Here's how the part is built. I have some questions about the finished solid (model axes, mm). A direction names the side the tool comes from. Give positions to 0.01 mm unless a question says otherwise; leave off trailing zeros. Loops run counter-clockwise (first coordinate to the right, second up) from the corner with the lowest first, then second, coordinate; pieces in that order, holes last. Notation, with made-up numbers: (-16.75, 8.5) - (6.25, 8.5) arc R24 cw to (6.25, 18.5) - close; hole circle Ø9 at (67.25, 31.25). An arc over 180 degrees is marked (long way). Use a Markdown table: item, result.
from build123d import *
from build123d.topology import SkipClean

# Parameters (mm, degrees)
SKETCH1_R           = 4.05
BOSS_EXTRUDE1_DEPTH = 5
SCALE1_SCALE        = 0.471698113
SKETCH2_R           = 1.910377358
BOSS_EXTRUDE3_DEPTH = 4.716981
SKETCH3_R           = 9.5
CUT_EXTRUDE1_DEPTH  = 35.525365892
SKETCH4_R           = 13.5
CUT_EXTRUDE2_DEPTH  = 35.525365892
SKETCH5_R           = 1.5
CUT_EXTRUDE3_DEPTH  = 35.525365892
FILLET1_R           = 5
BOSS_EXTRUDE4_START = 5
SKETCH6_R           = 9.5
SKETCH6_R_2         = 1.5
BOSS_EXTRUDE4_DEPTH = 5


with BuildPart() as part:
    # Sketch1 → Boss-Extrude1 (new, symmetric)
    with BuildSketch(Plane(origin=(0, 0, 0), x_dir=(1, 0, 0), z_dir=(0, 1, 0))):
        with BuildLine():
            Line((-38, 7.05), (38, 7.05))
            ThreePointArc((38, 7.05), (45.05, 0), (38, -7.05))
            Line((38, -7.05), (-38, -7.05))
            ThreePointArc((-38, -7.05), (-45.05, 0), (-38, 7.05))
        make_face()
        with Locations(Location((-38, 0, 0), (0, 0, 270))):
            Circle(SKETCH1_R, mode=Mode.SUBTRACT)
        with Locations(Location((38, 0, 0), (0, 0, 270))):
            Circle(SKETCH1_R, mode=Mode.SUBTRACT)
    extrude(amount=BOSS_EXTRUDE1_DEPTH, both=True)


with BuildPart() as part_1:
    # Scale1: scaled about (0, 0, 0)
    add(part.part.scale(SCALE1_SCALE))

    # Sketch2 → Boss-Extrude3 (add, through all)
    with BuildSketch(Plane(origin=(0, 2.358490566, 0), x_dir=(1, 0, 0), z_dir=(0, 1, 0))):
        with BuildLine():
            Line((8.163095128, 9.325471698), (-8.163095128, 9.325471698))
            ThreePointArc((-8.163095128, 9.325471698), (-31.424528302, 0), (-8.163095128, -9.325471698))
            Line((-8.163095128, -9.325471698), (8.163095128, -9.325471698))
            ThreePointArc((8.163095128, -9.325471698), (31.424528302, 0), (8.163095128, 9.325471698))
        make_face()
        with Locations(Location((-17.924528302, 0, 0), (0, 0, 270))):
            Circle(SKETCH2_R, mode=Mode.SUBTRACT)
        with Locations(Location((17.924528302, 0, 0), (0, 0, 270))):
            Circle(SKETCH2_R, mode=Mode.SUBTRACT)
    extrude(amount=-BOSS_EXTRUDE3_DEPTH)

    # Sketch3 → Cut-Extrude1 (cut, through all)
    with BuildSketch(Plane(origin=(0, 2.358490566, 0), x_dir=(1, 0, 0), z_dir=(0, 1, 0))):
        with Locations(Location((-17.924528302, 0, 0), (0, 0, 270))):
            Circle(SKETCH3_R)
        with Locations(Location((17.924528302, 0, 0), (0, 0, 270))):
            Circle(SKETCH3_R)
    extrude(amount=-CUT_EXTRUDE1_DEPTH, mode=Mode.SUBTRACT)

    # Sketch4 → Cut-Extrude2 (cut, through all)
    with BuildSketch(Plane(origin=(0, 2.358490566, 0), x_dir=(1, 0, 0), z_dir=(0, 1, 0))):
        with Locations((17.924528302, 0)):
            Circle(SKETCH4_R)
    extrude(amount=-CUT_EXTRUDE2_DEPTH, mode=Mode.SUBTRACT)

    # Sketch5 → Cut-Extrude3 (cut, through all)
    with BuildSketch(Plane(origin=(0, 2.358490566, 0), x_dir=(1, 0, 0), z_dir=(0, 1, 0))):
        with Locations(Location((0, 6.325471698, 0), (0, 0, 270))):
            Circle(SKETCH5_R)
        with Locations(Location((0, -6.325471698, 0), (0, 0, 270))):
            Circle(SKETCH5_R)
    extrude(amount=-CUT_EXTRUDE3_DEPTH, mode=Mode.SUBTRACT)

    # Fillet1
    # the kernel refuses this fillet: 5 mm, written as the material it takes off along each edge
    with BuildSketch(Plane(origin=(8.163095128, 22.922972313, -9.325471698), x_dir=(-0.47879135569736214, 0, 0.8779287201757795), z_dir=(0, -1, 0))) as fillet1_piece_1:
        with BuildLine():
            CenterArc((8.328082039, 4.827702878), FILLET1_R, 151.393506733, 103.521444362)
            Line((3.938438438, 7.221659656), (0, 0))
            ThreePointArc((0, 0), (3.51340961, 0.46520223), (7.02681922, 0))
        make_face()
    extrude(amount=45.845944493, mode=Mode.SUBTRACT)
    with BuildSketch(Plane(origin=(8.163095128, 22.922972313, 9.325471698), x_dir=(-1, 0, 0), z_dir=(0, -1, 0))) as fillet1_piece_2:
        with BuildLine():
            CenterArc((8.225792699, 5), FILLET1_R, 166.478555638, 103.521444362)
            ThreePointArc((3.364380301, 6.169046405), (2.090604549, 2.861788396), (0, 0))
            Line((0, 0), (8.225792699, 0))
        make_face()
    extrude(amount=45.845944493, mode=Mode.SUBTRACT)

    # Sketch6 → Boss-Extrude4 (add)
    with SkipClean():  # the faces are left unmerged after this step: merging them gives an invalid solid
        with BuildSketch(Plane(origin=(0, -2.358490566, 0), x_dir=(1, 0, 0), z_dir=(0, 1, 0)).offset(BOSS_EXTRUDE4_START)):
            with BuildLine():
                Line((-8.163095128, -9.325471698), (-0.062697571, -9.325471698))
                ThreePointArc((-0.062697571, -9.325471698), (3.864466293, -7.42020658), (4.798714827, -3.156425293))
                ThreePointArc((4.798714827, -3.156425293), (4.424528302, 0), (4.798714827, 3.156425293))
                ThreePointArc((4.798714827, 3.156425293), (3.864466293, 7.42020658), (-0.062697571, 9.325471698))
                Line((-0.062697571, 9.325471698), (-8.163095128, 9.325471698))
                ThreePointArc((-8.163095128, 9.325471698), (-31.424528302, 0), (-8.163095128, -9.325471698))
            make_face()
            with Locations(Location((-17.924528302, 0, 0), (0, 0, 270))):
                Circle(SKETCH6_R, mode=Mode.SUBTRACT)
            with Locations(Location((0, -6.325471698, 0), (0, 0, 270))):
                Circle(SKETCH6_R_2, mode=Mode.SUBTRACT)
            with Locations(Location((0, 6.325471698, 0), (0, 0, 270))):
                Circle(SKETCH6_R_2, mode=Mode.SUBTRACT)
        extrude(amount=-BOSS_EXTRUDE4_DEPTH)
    add(part_1.part.scale(1), mode=Mode.REPLACE)  # the faces are merged on a copy


solid = part_1.part
(1) On a 3-axis mill with a long thin cutter (end or side, diameter ignored), from which of +Z, -Z, +X, -X, +Y, -Y can I reach the whole of each face in a straight line? I mean faces 1 (the face through (-4, 0, 9.325)), 2 (the face through (-9, 2.642, 6)). Say none if no direction works.
A:
| item | result |
|---|---|
| face 1 | +Z, +X, +Y, -Y |
| face 2 | +Z, -Z, +X, -X, +Y |
(2) If I drill on line 1 (X direction, y = -0.3, z = 0); line 2 (Z direction, x = 1, y = -0.6); line 3 (X direction, y = 1.2, z = 8.25), over which ranges is the centre line in solid material (lowest first)?
A:
| item | result |
|---|---|
| line 1 | -31.42 to -27.42, -8.42 to 4.42 |
| line 2 | -9.21 to -7.44, -5.21 to 5.21, 7.44 to 9.21 |
| line 3 | -28.61 to -22.63, -13.21 to 3.04 |
(3) Will these pins go through, and if not, where does the flat tip stop? pin 1 (1 mm diameter, centred on x = -22, y = -1.5, fed in from +Z); pin 2 (2 mm diameter, centred on y = 0.5, z = -0.5, fed in from +X); pin 3 (1.5 mm diameter, centred on y = 0, z = 1.5, fed in from -X).
A:
| item | result |
|---|---|
| pin 1 | z = 13.02 |
| pin 2 | x = 4.51 |
| pin 3 | x = -31.4 |
(4) Suppose I cut it at D-D on z = 7.25. Write out the boundary of the cut face in (x, y).
A:
| item | result |
|---|---|
| outline | (-29.31, -2.36) - (-24.06, -2.36) - (-24.06, 2.64) - (-29.31, 2.64) - close; (-11.79, -2.36) - (-1.18, -2.36) - (-1.18, 2.64) - (-11.79, 2.64) - close; (1.18, -2.36) - (3.99, -2.36) - (3.99, 2.64) - (1.18, 2.64) - close |
(5) Suppose I cut it at B-B on x = 1. Write out the boundary of the cut face in (y, z), plus the area to 3 significant figures.
A:
| item | result |
|---|---|
| outline | (-2.36, -9.21) - (2.64, -9.21) - (2.64, -7.44) - (-2.36, -7.44) - close; (-2.36, -5.21) - (2.64, -5.21) - (2.64, 5.21) - (-2.36, 5.21) - close; (-2.36, 7.44) - (2.64, 7.44) - (2.64, 9.21) - (-2.36, 9.21) - close |
| area | 69.8 mm2 |
(6) Suppose I cut it at A-A on z = 0. Write out the boundary of the cut face in (x, y).
A:
| item | result |
|---|---|
| outline | (-31.42, -2.36) - (-27.42, -2.36) - (-27.42, 2.64) - (-31.42, 2.64) - close; (-8.42, -2.36) - (4.42, -2.36) - (4.42, 2.64) - (-8.42, 2.64) - close |
(7) Suppose I cut it at C-C on y = 1.35. Write out the boundary of the cut face in (x, z), plus the area to 3 significant figures.
A:
| item | result |
|---|---|
| outline | (-8.16, -9.33) - (-0.06, -9.33) arc R5 ccw to (4.8, -3.16) arc R13.5 cw to (4.8, 3.16) arc R5 ccw to (-0.06, 9.33) - (-8.16, 9.33) arc R13.5 ccw (long way) to start; hole circle Ø19 at (-17.92, 0); hole circle Ø3 at (0, -6.33); hole circle Ø3 at (0, 6.33) |
| area | 458 mm2 |
